Read the model definition and answer for the solid it produces. Units are mm, in the model's axes. Face numbers are marked on the shaded views. A direction names the side the tool comes from. Coordinates: 2 decimals unless noted, no trailing zeros. Write each loop counter-clockwise with the first axis right and the second up, starting at its lowest first coordinate (ties: lowest second). Pieces come first, ordered by that corner, then holes. Notation, with made-up numbers: M 9.5,89 L 37.5,89 A29 ccw 37.5,110 Z; hole C 21,45 d8. An arc over 180 degrees is marked long. Write item = value, one per line.
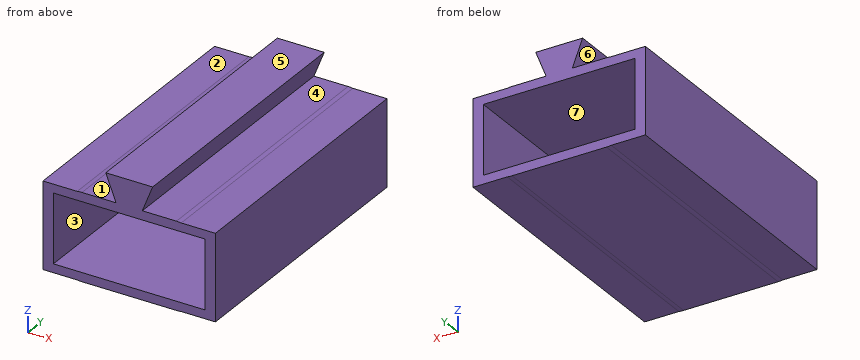
from build123d import *

# Parameters (mm, degrees)
F0_W      = 18.7
F0_H      = 38.5
F1_DEPTH  = 8
F2_R      = 2.5
F4_DEPTH  = 40
F7_DEPTH  = 40
F8_W      = 25
F8_H      = 12.5
F9_DEPTH  = 40
F10_W     = 22
F10_H     = 10
F11_DEPTH = 40


with BuildPart() as f1:
    # F0 (on Top) → F1 (new body)
    with BuildSketch(Plane.XY):
        Rectangle(F0_W, F0_H)
    extrude(amount=F1_DEPTH)

    # F2
    f2_edges = [f1.edges().sort_by_distance(p)[0] for p in [
        (9.35, 0, 8),
        (9.35, 0, 0),
        (-9.35, 0, 8),
        (-9.35, 0, 0),
    ]]
    fillet(f2_edges, radius=F2_R)


with BuildPart() as f4:
    # F3 (on face) → F4 (new body)
    with BuildSketch(Plane.XZ.offset(19.25)):
        with BuildLine():
            Line((-11.65, 5.5), (-11.65, 2.5))
            ThreePointArc((-11.65, 2.5), (-10.244113, -0.894113), (-6.85, -2.3))
            Line((-6.85, -2.3), (6.85, -2.3))
            ThreePointArc((6.85, -2.3), (10.244113, -0.894113), (11.65, 2.5))
            Line((11.65, 2.5), (11.65, 5.5))
            ThreePointArc((11.65, 5.5), (10.244113, 8.894113), (6.85, 10.3))
            Line((6.85, 10.3), (-6.85, 10.3))
            ThreePointArc((-6.85, 10.3), (-10.244113, 8.894113), (-11.65, 5.5))
        make_face()
        with BuildLine():
            Line((-6.85, 8.3), (6.85, 8.3))
            ThreePointArc((6.85, 8.3), (8.829899, 7.479899), (9.65, 5.5))
            Line((9.65, 5.5), (9.65, 2.5))
            ThreePointArc((9.65, 2.5), (8.829899, 0.520101), (6.85, -0.3))
            Line((6.85, -0.3), (-6.85, -0.3))
            ThreePointArc((-6.85, -0.3), (-8.829899, 0.520101), (-9.65, 2.5))
            Line((-9.65, 2.5), (-9.65, 5.5))
            ThreePointArc((-9.65, 5.5), (-8.829899, 7.479899), (-6.85, 8.3))
        make_face(mode=Mode.SUBTRACT)
    extrude(amount=-F4_DEPTH)

    # F6 (on face) → F7 (join)
    with BuildSketch(Plane.XZ.offset(19.25)):
        Polygon((3.4, 14.1), (1.9, 14.1), (-1.9, 14.1), (-3.4, 14.1), (-1.9, 10.3), (1.9, 10.3), align=None)
    extrude(amount=-F7_DEPTH)

    # F8 (on face) → F9 (join)
    with BuildSketch(Plane.XZ.offset(19.25)):
        with Locations((0, 4)):
            Rectangle(F8_W, F8_H)
    extrude(amount=-F9_DEPTH)

    # F10 (on face) → F11 (cut)
    with BuildSketch(Plane.XZ.offset(19.25)):
        with Locations((0, 4)):
            Rectangle(F10_W, F10_H)
    extrude(amount=-F11_DEPTH, mode=Mode.SUBTRACT)


solid = f4.part
Item 1: Find section A-A (z = 4.5). Determine the outline of the cut face in (x, y), and give its area (3 significant figures).
Worked answers:
outline = M -12.5,-19.25 L -11,-19.25 L -11,20.75 L -12.5,20.75 Z; M 11,-19.25 L 12.5,-19.25 L 12.5,20.75 L 11,20.75 Z
area = 120 mm²
Item 2: Consider line 1 along X through (y, z) = (-5.5, 3.5); line 2 along Z through (x, y) = (0, 17.5); line 3 along Z through (x, y) = (-4, 5). Determine where each line is inside the solid, lowest interval first. Write a range as from..to.
Worked answers:
line_1 = -12.5..-11, 11..12.5
line_2 = -2.3..-1, 9..14.1
line_3 = -2.3..-1, 9..10.3
Item 3: For a pull along X with two mould halves and no side action, classify the marked faces 5, 6 and 7 as released by +X, released by -X, zero draft, split by the parting line, or undercut.
Worked answers:
face_5 = zero draft
face_6 = released by -X
face_7 = undercut
Item 4: Find section B-B (x = -0.75). Determine the outline of the cut face in (y, z).
Worked answers:
outline = M -19.25,-2.3 L 20.75,-2.3 L 20.75,-1 L -19.25,-1 Z; M -19.25,9 L 20.75,9 L 20.75,14.1 L -19.25,14.1 Z
Item 5: Find section D-D (z = 12.75). Determine the outline of the cut face in (x, y), and give its area (3 significant figures).
Worked answers:
outline = M -2.87,-19.25 L 2.87,-19.25 L 2.87,20.75 L -2.87,20.75 Z
area = 229 mm²
Item 6: Flat-ended cylindrical pins translate along their axes: pin 1 (2 mm diameter, centred on x = 4, z = 0.5, fed in from +Y); pin 2 (1.5 mm diameter, centred on x = -9.5, y = 2, fed in from -Z); pin 3 (1.5 mm diameter, centred on x = -4.5, y = -4, fed in from +Z). Find the tip coordinate at first contact, or state that the pin passes through.
Worked answers:
pin_1 = through
pin_2 = -2.25
pin_3 = 10.3
Item 7: Which of the six approach directions +Z, -Z, +X, -X, +Y, -Y give full straight-line access (tool end or side, diameter ignored) to the marked faces 1, 2, 3 and 4?
Worked answers:
face_1 = -X, +Y, -Y
face_2 = +Z, -X, +Y, -Y
face_3 = +Y, -Y
face_4 = +X, +Y, -Y
Item 8: Find section C-C (y = 2). Determine the outline of the cut face in (x, z), and give its area (3 significant figures).
Worked answers:
outline = M -12.5,-2.25 L -7.54,-2.25 A4.8 ccw -6.85,-2.3 L 6.85,-2.3 A4.8 ccw 7.54,-2.25 L 12.5,-2.25 L 12.5,10.25 L 7.54,10.25 A4.8 ccw 6.85,10.3 L 1.9,10.3 L 3.4,14.1 L -3.4,14.1 L -1.9,10.3 L -6.85,10.3 A4.8 ccw -7.54,10.25 L -12.5,10.25 Z; hole M -11,-1 L 11,-1 L 11,9 L -11,9 Z
area = 114 mm²
